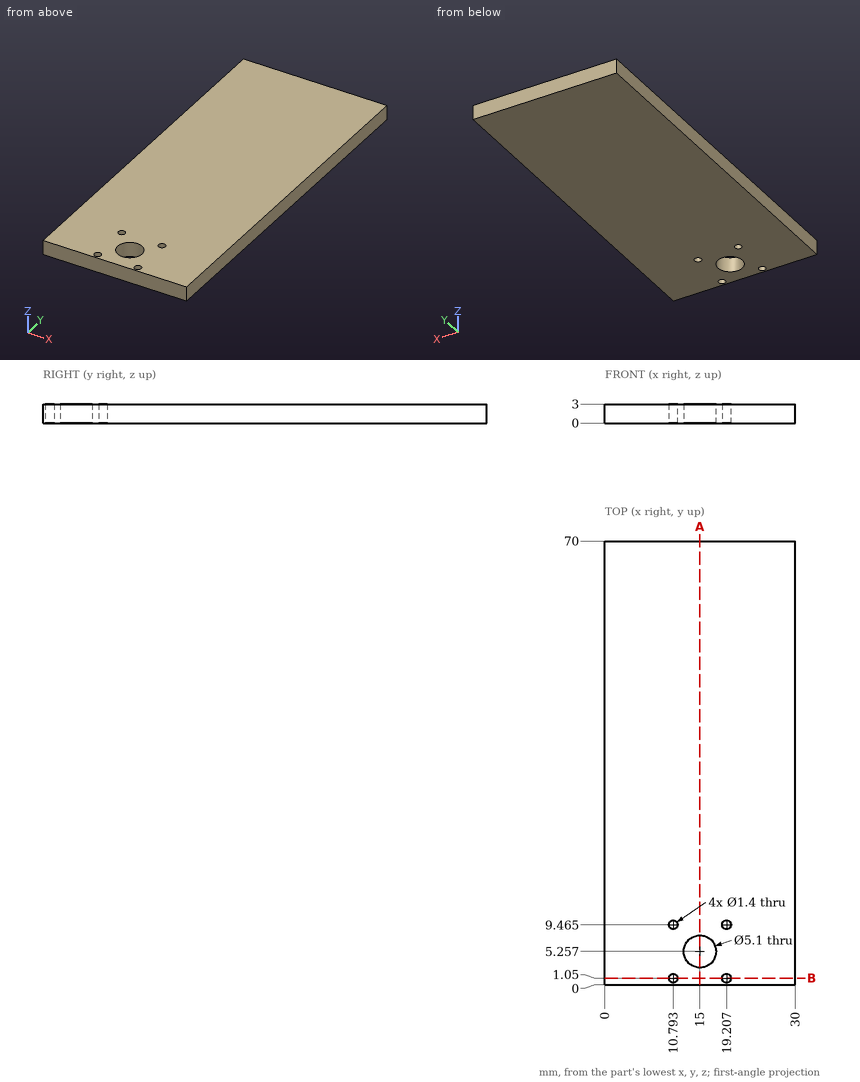
Input: dimensioned drawing with shaded views. Units: mm. Origin: part minimum x, y, z. Give positions to 0.01 mm unless a question says otherwise; leave off trailing zeros. Loops run counter-clockwise (first coordinate to the right, second up) from the corner with the lowest first, then second, coordinate; pieces in that order, holes last. Notation, with made-up numbers: (41.25, 74.5) -> (76.25, 74.5) arc R23 ccw to (76.25, 105.5) -> close; hole circle Ø10 at (54.5, 38.25). An arc over 180 degrees is marked (long way). Use a Markdown table: item, result. Add a question column.
1) Section query B-B, the plane y = 1.05. Return the cut outline in (x, z).
2) Section query A-A, the plane x = 15. Return the cut outline in (y, z).
3) Line query: line 1 along X through (y, z) = (9.5, 2.15); line 2 along Y through (x, z) = (19.5, 1.2) (1 decimal); line 3 along Y through (x, z) = (16, 1.75). Output: solid intervals per line, ascending. Write a range as [from, to].
4) First-contact query: pin 1 (8 mm diameter, centred on x = 7.5, y = 22, fed in from -Z); pin 2 (1.3 mm diameter, centred on x = 19.21, y = 1.05, fed in from -Z). Flat tips, straight axial feed; report the tip coordinate or a pass-through.
Numbers:
| question | item | result |
|---|---|---|
| 1 | outline | (0, 0) -> (10.09, 0) -> (10.09, 3) -> (0, 3) -> close; (11.49, 0) -> (18.51, 0) -> (18.51, 3) -> (11.49, 3) -> close; (19.91, 0) -> (30, 0) -> (30, 3) -> (19.91, 3) -> close |
| 2 | outline | (0, 0) -> (2.71, 0) -> (2.71, 3) -> (0, 3) -> close; (7.81, 0) -> (70, 0) -> (70, 3) -> (7.81, 3) -> close |
| 3 | line 1 | x = [0, 10.09], [11.49, 18.51], [19.91, 30] |
| 3 | line 2 | y = [0, 0.4], [1.7, 8.8], [10.1, 70] |
| 3 | line 3 | y = [0, 2.91], [7.6, 70] |
| 4 | pin 1 | stops at z = 0 |
| 4 | pin 2 | passes through |
